Work out the finished part from the listing and answer in its coordinate system (mm). A direction names the side the tool comes from. Coordinates: 2 decimals unless noted, no trailing zeros. Order: outer loops, then holes, each group sorted by start corner. A loop starts at its lowest first (then second) coordinate and runs counter-clockwise, first axis right, second up. Notation, with made-up numbers: M 82,-37.75 L 101,-37.75 A27 cw 101,-6.75 Z; hole C 34.25,89.5 d2. An arc over 180 degrees is marked long. Answer in a Markdown table with one row per item. Add a question column.
Item 1: The part is cut by section C-C (z = 4.75). State how many separate pieces and enclosed holes the cut face has, then the cut area to 3 significant figures.
Item 2: The mould has two halves that part along X. Classify faces 3 (the face through (0, 15, 12)), 4 (the face through (7.051, 22.395, 3.615)), 5 (the face through (58, 15, 12)), 6 (the face through (29, 30, 12)): released by +X, released by -X, zero draft, split by the parting line, or undercut.
Item 3: Consider line 1 (X direction, y = 25.25, z = 6); line 2 (Z direction, x = 51.7, y = 26.5); line 3 (X direction, y = 16.25, z = 3). Determine where each line is inside the solid, lowest interval first. Write a range as from..to.
Item 4: The part is cut by section A-A (x = 17.5). Write down the section's boundary in (y, z), then the cut area to 3 significant figures.
Item 5: Which of the six approach directions +Z, -Z, +X, -X, +Y, -Y give full straight-line access (tool end or side, diameter ignored) to faces 1 (the face through (50.2, 22.4, 21)), 2 (the face through (18.021, 18.966, 12.325))?
Item 6: The part is cut by section B-B (z = 11.5). Write down the section's boundary in (x, y).
Item 7: A flat-ended cylindrical pin translates along its axis: pin 1 Ø6.5 at (x, y) = (40.5, 15) entering from +Z. Find the tip coordinate at first contact, or state that the pin passes through.
from build123d import *

# Parameters (mm, degrees)
ESQUISSE1_W                                   = 58
ESQUISSE1_H                                   = 30
BOSS_EXTRU_1_DEPTH                            = 25
TROU_POUR_TARAUDAGE_POUR_TROU_TARAUD_M6_D     = 5
TROU_POUR_TARAUDAGE_POUR_TROU_TARAUD_M6_DEPTH = 15
TROU_POUR_TARAUDAGE_POUR_TROU_TARAUD_M6_TIP   = 1.502151548
DIAM_TRE_DU_PER_AGE_8_0_8_1_D                 = 8


with BuildPart() as part:
    # Esquisse1 → Boss.-Extru.1 (new body)
    with BuildSketch(Plane.XY):
        with Locations((29, 15)):
            Rectangle(ESQUISSE1_W, ESQUISSE1_H)
    extrude(amount=BOSS_EXTRU_1_DEPTH)

    # Trou pour taraudage pour trou taraudé M61
    with Locations(Plane(origin=(6.3, 30, 6), x_dir=(0, 0, 1), z_dir=(0, 1, 0))):
        with Locations((0, 0), (13, 0), (13, 45.4), (0, 45.4)):
            Hole(TROU_POUR_TARAUDAGE_POUR_TROU_TARAUD_M6_D / 2, depth=TROU_POUR_TARAUDAGE_POUR_TROU_TARAUD_M6_DEPTH)
            with Locations((0, 0, -(TROU_POUR_TARAUDAGE_POUR_TROU_TARAUD_M6_DEPTH + TROU_POUR_TARAUDAGE_POUR_TROU_TARAUD_M6_TIP / 2))):  # 118° drill point
                Cone(0, TROU_POUR_TARAUDAGE_POUR_TROU_TARAUD_M6_D / 2, TROU_POUR_TARAUDAGE_POUR_TROU_TARAUD_M6_TIP, mode=Mode.SUBTRACT)

    # Diamètre du perçage Ø8.0 (8)1 (through all)
    with Locations(Plane(origin=(17.5, 15, 25), x_dir=(1, 0, 0), z_dir=(0, 0, 1))):
        with Locations((0, 0), (23, 0)):
            Hole(DIAM_TRE_DU_PER_AGE_8_0_8_1_D / 2)


solid = part.part
Reply:
| question | item | result |
|---|---|---|
| 1 | separate pieces | 1 |
| 1 | enclosed holes | 2 |
| 1 | area | 1,510 mm2 |
| 2 | face 3 | released by -X |
| 2 | face 4 | undercut |
| 2 | face 5 | released by +X |
| 2 | face 6 | zero draft |
| 3 | line 1 | x = 0..3.8, 8.8..49.2, 54.2..58 |
| 3 | line 2 | z = 0..3.5, 8.5..16.5, 21.5..25 |
| 3 | line 3 | x = 0..13.7, 21.3..36.7, 44.3..58 |
| 4 | outline | M 0,0 L 11,0 L 11,25 L 0,25 Z; M 19,0 L 30,0 L 30,25 L 19,25 Z |
| 4 | area | 550 mm2 |
| 5 | face 1 | +Y |
| 5 | face 2 | +Z, -Z |
| 6 | outline | M 0,0 L 58,0 L 58,30 L 0,30 Z; hole C 17.5,15 d8; hole C 40.5,15 d8 |
| 7 | pin 1 | passes through |
